Read the model definition and answer for the solid it produces. Units are mm, in the model's axes. Face numbers are marked on the shaded views. A direction names the side the tool comes from. Give positions to 0.01 mm unless a question says otherwise; leave off trailing zeros. Loops run counter-clockwise (first coordinate to the right, second up) from the corner with the lowest first, then second, coordinate; pieces in that order, holes last. Notation, with made-up numbers: (-18, 34) -> (-5, 34) arc R38 cw to (-5, 72) -> close; hole circle Ø11 at (71, 76). An arc over 180 degrees is marked (long way). One line per item, written item: value. Start each with the question number.
Autodesk Inventor part; units mm, degrees
ref_plane "YZ Plane" through (0, 0, 0) normal (1, 0, 0) x (0, 1, 0)
ref_plane "XZ Plane" through (0, 0, 0) normal (0, 1, 0) x (-1, 0, 0)
ref_plane "XY Plane" through (0, 0, 0) normal (0, 0, 1) x (1, 0, 0)
sketch "Sketch1" plane through (0, 0, 0) normal (0, 1, 0) x (-1, 0, 0)
  line L0 (-10, -20.125) -> (10, -20.125)
  line L1 (10, -20.125) -> (10, 20.125)
  line L2 (10, 20.125) -> (-10, 20.125)
  line L3 (-10, 20.125) -> (-10, -20.125)
  line L4 (-10, -20.125) -> (10, 20.125) construction
  line L5 (10, -20.125) -> (-10, 20.125) construction
  line L6 (-11.5, -22) -> (11.5, -22)
  line L7 (11.5, -22) -> (11.5, 22)
  line L8 (11.5, 22) -> (-11.5, 22)
  line L9 (-11.5, 22) -> (-11.5, -22)
  line L10 (-11.5, -22) -> (11.5, 22) construction
  line L11 (11.5, -22) -> (-11.5, 22) construction
  line L12 (-10, 20.125) -> (-10, 22)
  line L13 (-10, -20.125) -> (-10, -22)
  point P0 (0, 0)
  dimension "d0" = 20
  dimension "d1" = 40.25
  dimension "d2" = 23
  dimension "d3" = 44
extrude "Extrusion1" add sketch "Sketch1" along normal blind 7 contours L0 L1 L2 L12 L8 L7 L6 L13
sketch "Sketch2" plane through (-11.5, 0, -22) normal (-1, 0, 0) x (0, 0, 1)
  line L0 (44, 0) -> (0, 0)
  line L1 (0, 0) -> (0, 22)
  line L2 (0, 22) -> (44, 22)
  line L3 (44, 22) -> (44, 0)
  point P0 (22, 0)
  dimension "d6" = 44
  dimension "d7" = 22
sketch "Sketch3" plane through (0, 7, 0) normal (0, 1, 0) x (1, 0, 0)
  line L0 (-10, -20.125) -> (-10, 20.125)
  line L1 (-10, 20.125) -> (10, 20.125)
  line L2 (10, 20.125) -> (10, 22)
  line L3 (10, 22) -> (-11.5, 22)
  line L4 (-11.5, 22) -> (-11.5, -22)
  line L5 (-11.5, -22) -> (10, -22)
  line L6 (10, -22) -> (10, -20.125)
  line L7 (10, -20.125) -> (-10, -20.125)
  line L8 (-10, 20.125) -> (-10, 22)
  point P0 (0, 0)
extrude "Extrusion2" add sketch "Sketch3" along normal blind 11 contours L7 L6 L5 L4 L3 L8 L0
sketch "Sketch4" plane through (0, 18, 0) normal (0, 1, 0) x (1, 0, 0)
  line L0 (10, -22) -> (10, -20.125)
  line L1 (-10, 22) -> (-11.5, 22)
  line L2 (10, -22) -> (-11.5, -22)
  line L3 (-11.5, -22) -> (-11.5, 22)
  line L4 (-11.5, 22) -> (10, 22)
  line L5 (10, 22) -> (10, -22)
  point P0 (0, 0)
extrude "Extrusion3" add sketch "Sketch4" along normal blind 4
sketch "Sketch5" plane through (0, 22, 0) normal (0, 1, 0) x (1, 0, 0)
  line L0 (10, 20.125) -> (10, 22)
  line L1 (10, 22) -> (-11.5, 22)
  line L2 (10, 22) -> (-11.5, 22)
  circle A0 centre (0, 10.2) radius 6.5
  circle A1 centre (0, 10.2) radius 9
  line L3 (0, 10.2) -> (-11.5, 10.2)
  line L4 (-11.5, 22) -> (-11.5, -22)
  line L5 (0, 10.2) -> (0, 14.2)
  line L6 (0, 14.2) -> (-11.5, 14.2)
  line L7 (0, 10.2) -> (0, 6.2)
  line L8 (0, 6.2) -> (-11.5, 6.2)
  line L9 (0, 6.2) -> (10, 6.2)
  line L10 (0, 14.2) -> (10, 14.2)
  line L11 (10, -22) -> (10, 22)
  line L12 (-11.5, -22) -> (10, -22)
  line L13 (10, -22) -> (10, 22)
  line L14 (10, 22) -> (-11.5, 22)
  line L15 (-11.5, 22) -> (-11.5, -22)
  point P0 (0, 0)
  point P1 (0, 22)
  point P2 (5.1235, 14.2)
  point P3 (8.0623, 14.2)
  point P4 (-8.0623, 14.2)
  point P5 (-5.1235, 14.2)
  point P6 (8.0623, 6.2)
  point P7 (5.1235, 6.2)
  point P8 (-5.1235, 6.2)
  point P9 (-8.0623, 6.2)
  dimension "d12" = 11.8
  dimension "d13" = 13
  dimension "d14" = 18
  dimension "d15" = 4
  dimension "d16" = 4
extrude "Extrusion4" add sketch "Sketch5" along normal blind 4 contours L10 A0 L6 A1 | A1 L8 A0 L9
fillet "Fillet1" radius 2 4 edges at (-5.1235, 24, -14.2) (5.1235, 24, -14.2) (-5.1235, 24, -6.2) (5.1235, 24, -6.2)
sketch "Sketch6" plane through (0, 22, 0) normal (0, 1, 0) x (1, 0, 0)
  line L0 (8.0623, 14.2) -> (6.0208, 14.2)
  arc A0 (4.6041, 14.7882) -> (6.0208, 14.2) centre (6.0208, 16.2) ccw
  arc A1 (4.6041, 14.7882) -> (-4.6041, 14.7882) centre (0, 10.2) ccw
  arc A2 (-6.0208, 14.2) -> (-4.6041, 14.7882) centre (-6.0208, 16.2) ccw
  line L1 (-6.0208, 14.2) -> (-8.0623, 14.2)
  arc A3 (8.0623, 14.2) -> (-8.0623, 14.2) centre (0, 10.2) ccw
  line L2 (6.0208, 6.2) -> (8.0623, 6.2)
  arc A4 (-8.0623, 6.2) -> (8.0623, 6.2) centre (0, 10.2) ccw
  line L3 (-8.0623, 6.2) -> (-6.0208, 6.2)
  arc A5 (-4.6041, 5.6118) -> (-6.0208, 6.2) centre (-6.0208, 4.2) ccw
  arc A6 (-4.6041, 5.6118) -> (4.6041, 5.6118) centre (0, 10.2) ccw
  arc A7 (6.0208, 6.2) -> (4.6041, 5.6118) centre (6.0208, 4.2) ccw
  line L4 (-11.5, -22) -> (10, -22)
  line L5 (10, -22) -> (10, 22)
  line L6 (10, 22) -> (-11.5, 22)
  line L7 (-11.5, 22) -> (-11.5, -22)
  arc A8 (6.0208, 6.2) -> (4.6041, 5.6118) centre (6.0208, 4.2) ccw
  arc A9 (-4.6041, 5.6118) -> (4.6041, 5.6118) centre (0, 10.2) ccw
  arc A10 (-4.6041, 5.6118) -> (-6.0208, 6.2) centre (-6.0208, 4.2) ccw
  line L8 (-6.0208, 6.2) -> (-8.0623, 6.2)
  arc A11 (-8.0623, 6.2) -> (8.0623, 6.2) centre (0, 10.2) ccw
  line L9 (8.0623, 6.2) -> (6.0208, 6.2)
  arc A12 (4.6041, 14.7882) -> (6.0208, 14.2) centre (6.0208, 16.2) ccw
  line L10 (6.0208, 14.2) -> (8.0623, 14.2)
  arc A13 (8.0623, 14.2) -> (-8.0623, 14.2) centre (0, 10.2) ccw
  line L11 (-8.0623, 14.2) -> (-6.0208, 14.2)
  arc A14 (-6.0208, 14.2) -> (-4.6041, 14.7882) centre (-6.0208, 16.2) ccw
  arc A15 (4.6041, 14.7882) -> (-4.6041, 14.7882) centre (0, 10.2) ccw
  line L12 (-8.0623, 6.2) -> (-11.5, 6.2)
  line L13 (-8.0623, 14.2) -> (-11.5, 14.2)
  line L14 (-11.5, 22) -> (-11.5, -22)
  line L15 (8.0623, 6.2) -> (10, 6.2)
  line L16 (8.0623, 14.2) -> (10, 14.2)
  circle A16 centre (0, 10.2) radius 12.5
  circle A17 centre (0, 10.2) radius 1.6
  point P0 (0, 0)
  point P1 (-11.5, 5.301)
  point P2 (10, 2.7)
  point P3 (10, 17.7)
  point P4 (-11.5, 15.099)
  dimension "d20" = 25
  dimension "d21" = 3.2
extrude "Extrusion5" add sketch "Sketch6" along normal up to surface (4 mm away) contours A3 L13 L7 A16 L6 L5 L16 | L5 A16 L7 L12 A4 L15 | L6 A16
extrude "Extrusion6" cut sketch "Sketch6" against normal blind 10 contours A17
sketch "Sketch7" plane through (10, 0, -20.125) normal (1, 0, 0) x (0, 0, -1)
  line L0 (0, 0) -> (1.875, 0)
  line L1 (1.875, 0) -> (1.875, 7)
  line L2 (0, 7) -> (1.875, 7)
  line L3 (0, 0) -> (0, 7)
  line L4 (-42.125, 0) -> (-40.25, 0)
  line L5 (-40.25, 0) -> (-40.25, 18)
  line L6 (-40.25, 18) -> (1.875, 18)
  line L7 (1.875, 18) -> (1.875, 22)
  line L8 (-2.425, 22) -> (1.875, 22)
  line L9 (-2.425, 22) -> (-2.425, 26)
  line L10 (-2.425, 26) -> (-5.925, 26)
  line L11 (-5.925, 22) -> (-5.925, 26)
  line L12 (-13.925, 22) -> (-5.925, 22)
  line L13 (-13.925, 22) -> (-13.925, 26)
  line L14 (-13.925, 26) -> (-17.425, 26)
  line L15 (-17.425, 22) -> (-17.425, 26)
  line L16 (-42.125, 22) -> (-17.425, 22)
  line L17 (-42.125, 0) -> (-42.125, 22)
  line L18 (1.875, 0) -> (1.875, 7)
  circle A0 centre (1.875, 3.5) radius 1.875
  line L19 (-42.125, 0) -> (-42.125, 22)
  circle A1 centre (-42.125, 3.5) radius 1.875
  point P0 (-20.125, 0)
  point P1 (-42.125, 5.375)
  point P2 (-42.125, 1.625)
  point P3 (1.875, 5.375)
  point P4 (1.875, 1.625)
  dimension "d26" = 3.75
  dimension "d27" = 3.75
extrude "Extrusion7" add sketch "Sketch7" against normal up to surface (21.5 mm away) contours L1 A0 | A1 L17 picked at (2.2647, 3.9886) picked at (-43.0085, 3.7216)
sketch "Sketch8" plane through (10, 0, -20.125) normal (1, 0, 0) x (0, 0, -1)
  line L0 (0, 0) -> (1.875, 0)
  line L1 (1.875, 0) -> (1.875, 1.625)
  arc A0 (1.875, 1.625) -> (1.875, 5.375) centre (1.875, 3.5) ccw
  line L2 (1.875, 5.375) -> (1.875, 7)
  line L3 (0, 7) -> (1.875, 7)
  line L4 (0, 0) -> (0, 7)
  line L5 (-42.125, 0) -> (-40.25, 0)
  line L6 (-40.25, 0) -> (-40.25, 18)
  line L7 (-40.25, 18) -> (1.875, 18)
  line L8 (1.875, 18) -> (1.875, 22)
  line L9 (-2.425, 22) -> (1.875, 22)
  line L10 (-2.425, 22) -> (-2.425, 26)
  line L11 (-2.425, 26) -> (-5.925, 26)
  line L12 (-5.925, 22) -> (-5.925, 26)
  line L13 (-13.925, 22) -> (-5.925, 22)
  line L14 (-13.925, 22) -> (-13.925, 26)
  line L15 (-13.925, 26) -> (-17.425, 26)
  line L16 (-17.425, 22) -> (-17.425, 26)
  line L17 (-42.125, 22) -> (-17.425, 22)
  line L18 (-42.125, 5.375) -> (-42.125, 22)
  arc A1 (-42.125, 5.375) -> (-42.125, 1.625) centre (-42.125, 3.5) ccw
  line L19 (-42.125, 0) -> (-42.125, 1.625)
  circle A2 centre (-42.125, 3.5) radius 1
  circle A3 centre (1.875, 3.5) radius 1
  point P0 (-20.125, 0)
  dimension "d30" = 2
  dimension "d31" = 2
extrude "Extrusion8" cut sketch "Sketch8" against normal blind 6 contours A2 | A3
sketch "Sketch9" plane through (10, 0, 22) normal (1, 0, 0) x (0, 0, -1)
  line L0 (1.875, 0) -> (1.875, 18)
  line L1 (44, 0) -> (0, 0)
  line L2 (1.875, 18) -> (1.675, 18)
  line L3 (1.675, 18) -> (1.675, 0)
  line L4 (1.675, 0) -> (1.875, 0)
  line L5 (1.875, 0) -> (1.875, 18)
  line L6 (42.125, 0) -> (42.125, 7)
  line L7 (42.125, 0) -> (44, 0)
  line L8 (42.125, 7) -> (42.325, 7)
  line L9 (42.325, 7) -> (42.325, 0)
  line L10 (42.325, 0) -> (42.125, 0)
  line L11 (42.125, 0) -> (42.125, 7)
  point P0 (22, 0)
  dimension "d34" = 0.2
  dimension "d35" = 0.2
extrude "Extrusion9" cut sketch "Sketch9" against normal up to surface (20 mm away)
sketch "Sketch10" plane through (-10, 7, -22) normal (1, 0, 0) x (0, 0, -1)
  line L0 (-42.325, -7) -> (-1.675, -7)
  line L1 (-1.675, 0) -> (-1.675, -7)
  line L2 (0, 0) -> (-1.675, 0)
  line L3 (0, 0) -> (0, 11)
  line L4 (-42.325, 11) -> (0, 11)
  line L5 (-42.325, -7) -> (-42.325, 11)
  line L6 (0, 0) -> (-1.675, 0)
  line L7 (-1.675, 0) -> (-1.675, 11)
  line L8 (-1.675, 11) -> (0, 11)
  line L9 (0, 11) -> (0, 0)
  point P0 (-22, -7)
extrude "Extrusion10" add sketch "Sketch10" along normal blind 5 contours L7 L4 L3 L2
sketch "Sketch11" plane through (0, 18, 0) normal (0, -1, 0) x (1, 0, 0)
  circle A0 centre (0, 8.6768) radius 1.5
  point P0 (0, 0)
  dimension "d40" = 3
extrude "Extrusion11" cut sketch "Sketch11" against normal blind 5
properties part number "Gripper3overhead_3DPrint"
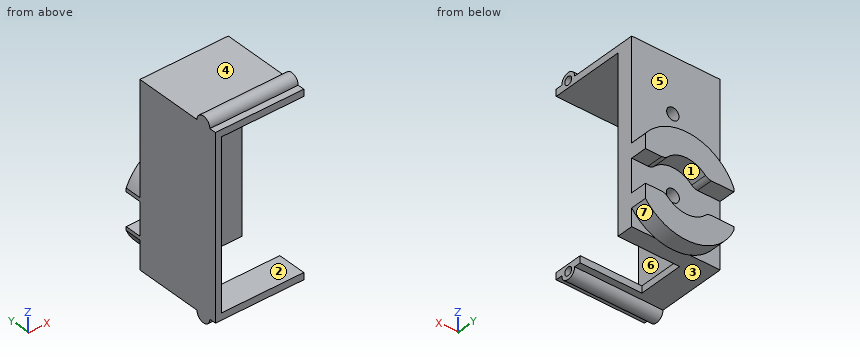
Item 1: Consider L1, parallel to Z at x = 0, y = 19.7; L2, parallel to Z at x = -2.5, y = 3.5 (3 decimals); L3, parallel to Z at x = 0.5, y = 6 (3 decimals). Determine where each line is inside the solid, lowest interval first. Write a range as [from, to].
Item 2: Section B-B, the plane y = 3.5 is taken. Determine the outline of the cut face in (x, z) (3 decimals), plus the area to 3 significant figures.
Item 3: Determine the mould class of the marked faces 5, 6 and 7 for opening direction Z: pulls with the +Z half, pulls with the -Z half, needs draft (parallel to the pull), parting line crosses it, or undercut.
Item 4: Section C-C, the plane x = 2.75 is taken. Determine the outline of the cut face in (y, z) (3 decimals).
Item 5: Flat-ended cylindrical pins translate along their axes: pin 1 (1 mm diameter, centred on x = -8, z = 13, fed in from +Y); pin 2 (2 mm diameter, centred on x = -9, y = 25, fed in from +Z); pin 3 (10 mm diameter, centred on y = 9, z = -15.5, fed in from +X); pin 4 (2.5 mm diameter, centred on y = 3.5, z = -22, fed in from +X). Find the tip coordinate at first contact, or state that the pin passes through.
Item 6: Section D-D, the plane z = 1 is taken. Determine the outline of the cut face in (x, y).
Item 7: For the marked faces 1, 2, 3 and 4, determine the directions among +Z, -Z, +X, -X, +Y, -Y from which every point of the face is accessible in a straight line to the end or side of a thin tool.
Item 8: Section A-A, the plane z = -10.2 is taken. Determine the outline of the cut face in (x, y), plus the area to 3 significant figures.
Computed values:
1. L1: [-22, -11.8], [-8.6, 7.18], [10.18, 22]
1. L2: [-23.875, -20.325], [20.325, 23.875]
1. L3: [-22, -20.325], [20.325, 22]
2. outline: (-11.5, -23.875) -> (10, -23.875) -> (10, -23) -> (4, -23) -> (4, -21) -> (10, -21) -> (10, -20.325) -> (-10, -20.325) -> (-10, 20.325) -> (10, 20.325) -> (10, 21) -> (4, 21) -> (4, 23) -> (10, 23) -> (10, 23.875) -> (-11.5, 23.875) -> close
2. area: 190 mm²
3. face 5: needs draft
3. face 6: undercut
3. face 7: pulls with the -Z half
4. outline: (0, -22) -> (1.625, -22) arc R1.875 ccw to (5.375, -22) -> (7, -22) -> (7, -20.325) -> (0, -20.325) -> close; (0, 20.325) -> (18, 20.325) -> (18, -22) -> (22, -22) -> (22, -22.394) -> (26, -22.394) -> (26, -16.09) -> (22, -16.09) -> (22, -4.31) -> (26, -4.31) -> (26, 1.994) -> (22, 1.994) -> (22, 22) -> (5.375, 22) arc R1.875 ccw to (1.625, 22) -> (0, 22) -> close
5. pin 1: y = 22
5. pin 2: z = -0.6
5. pin 3: x = -5
5. pin 4: x = 10
6. outline: (-11.5, 0) -> (-10, 0) -> (-10, 18) -> (10, 18) -> (10, 22) -> (5.55, 22) -> (5.55, 26) -> (-5.55, 26) -> (-5.55, 22) -> (-11.5, 22) -> close
7. face 1: +Y
7. face 2: +X, -Y
7. face 3: -Z, +X, -X
7. face 4: +Z, +X, -X, +Y
8. outline: (-11.5, 0) -> (-10, 0) -> (-10, 18) -> (-1.6, 18) -> (-1.6, 22) -> (-11.5, 22) -> close; (1.6, 18) -> (10, 18) -> (10, 22) -> (1.6, 22) -> close
8. area: 100 mm²
